Part model, mm, in its own coordinate system. A direction names the side the tool comes from. Round coordinates to 2 decimals unless told otherwise and drop trailing zeros. Loops run counter-clockwise (first coordinate to the right, second up) from the corner with the lowest first, then second, coordinate; pieces in that order, holes last. Notation, with made-up numbers: M -22,-3 L 26,-3 A38 cw 26,35 Z; hole C -13,82 d4. An arc over 180 degrees is marked long. Write each question's results on one line, items separated by ' | '.
from build123d import *

# Parameters (mm, degrees)
BOSS_EXTRUDE1_DEPTH = 20
SKETCH2_R           = 35
BOSS_EXTRUDE2_DEPTH = 40
SKETCH3_W           = 30
SKETCH3_H           = 25
CUT_EXTRUDE1_DEPTH  = 128
SKETCH4_W           = 89.4427191
SKETCH4_H           = 25
CUT_EXTRUDE2_DEPTH  = 15
BOSS_EXTRUDE3_DEPTH = 20


with BuildPart() as part:
    # Sketch1 → Boss-Extrude1 (new body)
    with BuildSketch(Plane(origin=(0, 0, 0), x_dir=(1, 0, 0), z_dir=(0, 1, 0))):
        with BuildLine():
            Line((-44.72135955, -40), (44.72135955, -40))
            ThreePointArc((44.72135955, -40), (60, 0), (44.72135955, 40))
            Line((44.72135955, 40), (-44.72135955, 40))
            ThreePointArc((-44.72135955, 40), (-60, 0), (-44.72135955, -40))
        make_face()
    extrude(amount=BOSS_EXTRUDE1_DEPTH)

    # Sketch2 → Boss-Extrude2 (add)
    with BuildSketch(Plane(origin=(0, 20, 0), x_dir=(1, 0, 0), z_dir=(0, 1, 0))):
        with Locations(Location((0, 0, 0), (0, 0, 270))):
            Circle(SKETCH2_R)
    extrude(amount=BOSS_EXTRUDE2_DEPTH)

    # Sketch3 → Cut-Extrude1 (cut)
    with BuildSketch(Plane.XY.offset(40)):
        with Locations((0, 22.5)):
            Rectangle(SKETCH3_W, SKETCH3_H)
    extrude(amount=-CUT_EXTRUDE1_DEPTH, mode=Mode.SUBTRACT)

    # Sketch4 → Cut-Extrude2 (cut)
    with BuildSketch(Plane.XY.offset(40)):
        with Locations((0, 32.5)):
            Rectangle(SKETCH4_W, SKETCH4_H)
    cut_extrude2 = extrude(amount=-CUT_EXTRUDE2_DEPTH, mode=Mode.SUBTRACT)

    # Mirror1: Cut-Extrude2 across plane
    add(cut_extrude2.mirror(Plane.XY), mode=Mode.SUBTRACT)

    # Sketch6 → Boss-Extrude3 (add)
    with BuildSketch(Plane(origin=(0, 60, 0), x_dir=(1, 0, 0), z_dir=(0, 1, 0))):
        with BuildLine():
            ThreePointArc((20, 28.722813233), (0, 35), (-20, 28.722813233))
            Line((-20, 28.722813233), (-20, 15))
            ThreePointArc((-20, 15), (0, 25), (20, 15))
            Line((20, 15), (20, 28.722813233))
        make_face()
        with BuildLine():
            Line((-20, -15), (-20, -28.722813233))
            ThreePointArc((-20, -28.722813233), (0, -35), (20, -28.722813233))
            Line((20, -28.722813233), (20, -15))
            ThreePointArc((20, -15), (0, -25), (-20, -15))
        make_face()
    extrude(amount=BOSS_EXTRUDE3_DEPTH)


solid = part.part
Item 1: Band-saw the part on D-D on z = 0. Give the cut face in (x, y), and give its area (3 significant figures).
Filled sheet:
outline: M -60,0 L 60,0 L 60,20 L 35,20 L 35,60 L -35,60 L -35,20 L -60,20 Z; hole M -15,10 L 15,10 L 15,35 L -15,35 Z | area: 4,450 mm^2
Item 2: Band-saw the part on A-A on y = 17.5. Give the cut face in (x, z), and give its area (3 significant figures).
Filled sheet:
outline: M -44.72,-40 L -15,-40 L -15,40 L -44.72,40 A60 ccw Z; M 15,-40 L 44.72,-40 A60 ccw 44.72,40 L 15,40 Z | area: 6,430 mm^2
Item 3: Band-saw the part on B-B on x = 0. Give the cut face in (y, z).
Filled sheet:
outline: M 0,-40 L 10,-40 L 10,40 L 0,40 Z; M 35,-25 L 45,-25 L 45,-35 L 80,-35 L 80,-25 L 60,-25 L 60,25 L 80,25 L 80,35 L 45,35 L 45,25 L 35,25 Z
Item 4: Wall check: L1, parallel to Y at x = 10.5, z = 26; L2, parallel to Y at x = 2, z = 19.5; L3, parallel to Y at x = -55, z = 6.5. Give the ranges that are in metal, low to high.
Filled sheet:
L1: 0 to 10, 45 to 80 | L2: 0 to 10, 35 to 60 | L3: 0 to 20
Item 5: Band-saw the part on C-C on z = -30.5. Give the cut face in (x, y).
Filled sheet:
outline: M -51.67,0 L 51.67,0 L 51.67,20 L 15,20 L 15,10 L -15,10 L -15,20 L -51.67,20 Z; M -17.17,45 L 17.17,45 L 17.17,80 L -17.17,80 Z
Item 6: Two-plate mould, pull along Z, no slides. Class faces 4 (the cylindrical face through (0, 70, -25)), 5 (the flat face through (1, 8, -40)), 6 (the flat face through (0, 35, 0)): +Z half, -Z half, draft (parallel to the pull), parting line (faces both ways), or undercut.
Filled sheet:
face 4: undercut | face 5: -Z half | face 6: draft
Item 7: Which spindle directions (+Z, -Z, +X, -X, +Y, -Y) get a long thin tool onto all of the face, cutting with end or side? Do faces 1 (the flat face through (-0.3, 35.5, -25)), 2 (the flat face through (0, 10, 1)), 3 (the flat face through (-0.3, 35.5, 25)). Say none if no direction does.
Filled sheet:
face 1: -Z, +X, -X | face 2: +Z, -Z | face 3: +Z, +X, -X
Item 8: Drop flat-ended pins along their axis: P1, Ø7, axis at y = 72.5, z = -24.5, coming from the -X side; P2, Ø12.5, axis at x = -0.5, y = 35.5, coming from the -Z side; P3, Ø20, axis at x = 3.5, y = 38, coming from the +Z side; P4, Ø5, axis at x = 0.5, z = 29.5, coming from the -Y side. Give the stop position or say it passes through.
Filled sheet:
P1: x = -20 | P2: z = -25 | P3: z = 35 | P4: y = 0
